Print and shaded views of the part. All mm, measured from the part's lowest x, y and z. A direction names the side the tool comes from. Round coordinates to 2 decimals unless told otherwise and drop trailing zeros. Write each loop counter-clockwise with the first axis right and the second up, starting at its lowest first coordinate (ties: lowest second). Pieces come first, ordered by that corner, then holes. Notation, with made-up numbers: (-10.75, -32) - (41.25, -32) arc R24 cw to (41.25, -8) - close; hole circle Ø6 at (-10.5, 75.5). An arc over 180 degrees is marked (long way). Put each result on its own line as item: value. Start each with the question number.
Item 1: Drill centre lines: line 1 (Y direction, x = 150, z = 54.75); line 2 (Y direction, x = 60.5, z = 52); line 3 (X direction, y = 80.5, z = 44.5). Where is each one in solid material? Low to high. Write a range as from..to.
Item 2: Cut at A-A (z = 51). Give the cut face in (x, y).
Item 3: Cut at C-C (y = 56). Give the cut face in (x, z), and give its area (3 significant figures).
Item 4: Pin check, flat tips, straight feed: pin 1 Ø1 at (x, y) = (59.5, 25) entering from +Z; pin 2 Ø6 at (x, z) = (24, 28) entering from +Y; pin 3 Ø1.5 at (x, z) = (89.5, 23) entering from -Y. Stop position of each tip, or through.
Item 5: 3-axis set-ups, long thin cutter, end or side, ignore diameter. For the marked faces 1, 2, 3, 4 and 5: which of +Z, -Z, +X, -X, +Y, -Y reach the whole face in a straight line?
Item 6: Mould opens along Y. For the marked faces 6, 7 and 8 say: released by +Y, released by -Y, zero draft, split by the parting line, or undercut.
Item 7: Cut at D-D (x = 58). Give the cut face in (y, z), and give its area (3 significant figures).
Item 8: Cut at B-B (x = 150). Give the cut face in (y, z).
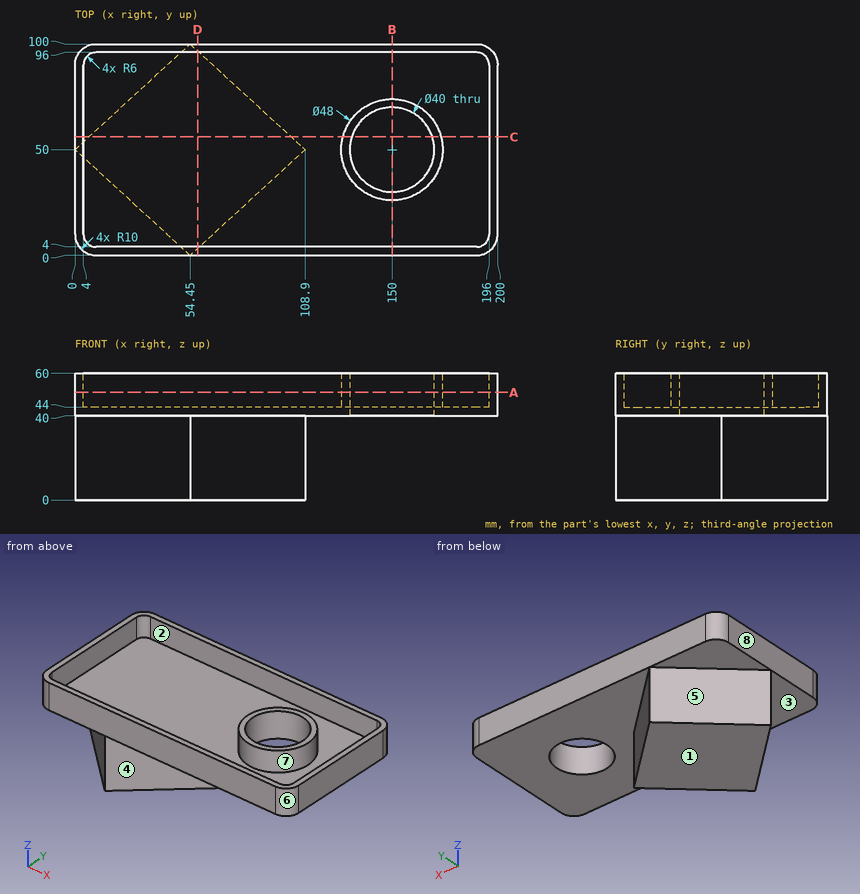
Output values:
1. line 1: 0..4, 26..30, 70..74, 96..100
1. line 2: 0..4, 96..100
1. line 3: 0..4, 196..200
2. outline: (0, 10) arc R10 ccw to (10, 0) - (190, 0) arc R10 ccw to (200, 10) - (200, 90) arc R10 ccw to (190, 100) - (10, 100) arc R10 ccw to (0, 90) - close; circle Ø48 at (150, 50); hole (4, 10) arc R6 ccw to (10, 4) - (190, 4) arc R6 ccw to (196, 10) - (196, 90) arc R6 ccw to (190, 96) - (10, 96) arc R6 ccw to (4, 90) - close; hole circle Ø40 at (150, 50)
3. outline: (0, 40) - (6.53, 40) - (6.53, 0) - (102.37, 0) - (102.37, 40) - (130.92, 40) - (130.92, 60) - (126.76, 60) - (126.76, 44) - (4, 44) - (4, 60) - (0, 60) - close; (169.08, 40) - (200, 40) - (200, 60) - (196, 60) - (196, 44) - (173.24, 44) - (173.24, 60) - (169.08, 60) - close
3. area: 4,740 mm2
4. pin 1: z = 44
4. pin 2: y = 74.79
4. pin 3: y = 31.5
5. face 1: -Z, +X, -X, +Y, -Y
5. face 2: +Z
5. face 3: -Z, -X, -Y
5. face 4: -Z, +X, -Y
5. face 5: -Z, -X, +Y
6. face 6: released by -Y
6. face 7: undercut
6. face 8: zero draft
7. outline: (0, 40) - (3.26, 40) - (3.26, 0) - (96.74, 0) - (96.74, 40) - (100, 40) - (100, 60) - (96, 60) - (96, 44) - (4, 44) - (4, 60) - (0, 60) - close
7. area: 4,270 mm2
8. outline: (0, 40) - (30, 40) - (30, 60) - (26, 60) - (26, 44) - (4, 44) - (4, 60) - (0, 60) - close; (70, 40) - (100, 40) - (100, 60) - (96, 60) - (96, 44) - (74, 44) - (74, 60) - (70, 60) - close
